Geometry: final body of the model. Coordinates: model frame, mm. Give positions to 0.01 mm unless a question says otherwise; leave off trailing zeros. Write each loop counter-clockwise with the first axis right and the second up, starting at its lowest first coordinate (ties: lowest second). Pieces come first, ordered by that corner, then holes. Notation, with made-up numbers: M -6,-28 L 34,-28 A25 cw 34,2 Z; hole C -25.5,-40 d2. An arc over 180 degrees is marked long. Use one line per item in the form item = value. Start each with the question number.
Item 1: Contact query for a flat-ended pin moving along its axis: P1, Ø5.5, axis at x = 0, y = 0, coming from the +Z side. Output: stop coordinate, or through.
Item 2: Section query A-A on x = 0. Return loops of the section in (y, z).
Item 3: Material intervals for line 1 along Y through (x, z) = (0, -0.7); line 2 along X through (y, z) = (80, -0.35); line 3 along X through (y, z) = (66, 0.75), sorted ascending. Write a range as from..to.
Item 4: Section query C-C on y = 30. Return loops of the section in (x, z), then the cut area to 3 significant figures.
Item 5: Section query B-B on z = 0.95. Return loops of the section in (x, y), then the cut area to 3 significant figures.
Autodesk Inventor part; units mm, degrees
ref_plane "YZ Plane" through (0, 0, 0) normal (1, 0, 0) x (0, 1, 0)
ref_plane "XZ Plane" through (0, 0, 0) normal (0, 1, 0) x (-1, 0, 0)
ref_plane "XY Plane" through (0, 0, 0) normal (0, 0, 1) x (1, 0, 0)
sketch "Sketch1" plane through (0, 0, 0) normal (0, 0, 1) x (1, 0, 0)
  circle A0 centre (0, 0) radius 6
  line L0 (0, 0) -> (0, 80) construction
  line L1 (6, 0) -> (6, 80)
  line L2 (-6, 80) -> (-6, 0)
  arc A1 (-6, 0) -> (6, 0) centre (0, 0) ccw
  arc A2 (6, 80) -> (-6, 80) centre (0, 80) ccw
  point P0 (0, 40)
  dimension "d0" = 12
  dimension "d1" = 12
  dimension "d2" = 80
extrude "Extrusion1" add sketch "Sketch1" along normal mid plane 2.8
sketch "Sketch2" plane through (0, 0, 1.4) normal (0, 0, 1) x (1, 0, 0)
  arc A0 (6, 80) -> (-6, 80) centre (0, 80) ccw construction
  arc A1 (-6, 0) -> (6, 0) centre (0, 0) ccw construction
  circle A2 centre (0, 0) radius 1.75
  circle A3 centre (0, 80) radius 1.75
  line L0 (-1.5, 64.9) -> (1.5, 64.9)
  line L1 (1.5, 64.9) -> (1.5, 70.1)
  line L2 (1.5, 70.1) -> (-1.5, 70.1)
  line L3 (-1.5, 70.1) -> (-1.5, 64.9)
  circle A4 centre (0, 30) radius 1.75
  line L4 (-1.5, 9.9) -> (1.5, 9.9)
  line L5 (1.5, 9.9) -> (1.5, 18.1)
  line L6 (1.5, 18.1) -> (-1.5, 18.1)
  line L7 (-1.5, 18.1) -> (-1.5, 9.9)
  point P0 (0, 9.9)
  point P1 (0, 64.9)
  point P2 (1.5, 14)
  point P3 (1.5, 67.5)
  dimension "d8" = 3.5
  dimension "d9" = 3.5
  dimension "d12" = 3
  dimension "d13" = 8.2
  dimension "d16" = 5.2
  dimension "d18" = 14
  dimension "d19" = 30
  dimension "d20" = 12.5
extrude "Extrusion2" cut sketch "Sketch2" against normal through all
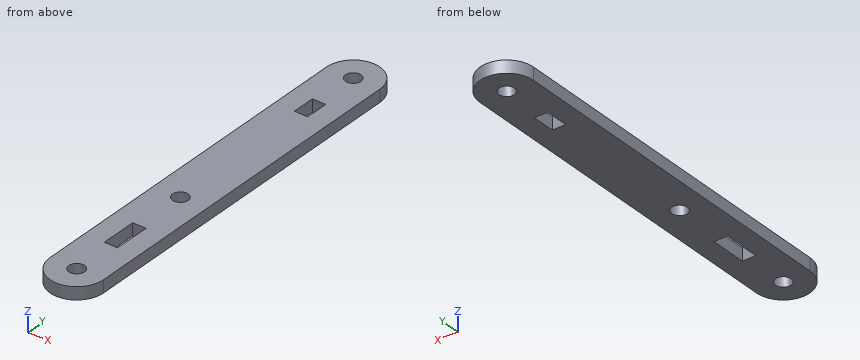
Answer sheet:
q1.P1 = 1.4
q2.outline = M -6,-1.4 L -1.75,-1.4 L -1.75,1.4 L -6,1.4 Z; M 1.75,-1.4 L 9.9,-1.4 L 9.9,1.4 L 1.75,1.4 Z; M 18.1,-1.4 L 28.25,-1.4 L 28.25,1.4 L 18.1,1.4 Z; M 31.75,-1.4 L 64.9,-1.4 L 64.9,1.4 L 31.75,1.4 Z; M 70.1,-1.4 L 78.25,-1.4 L 78.25,1.4 L 70.1,1.4 Z; M 81.75,-1.4 L 86,-1.4 L 86,1.4 L 81.75,1.4 Z
q3.line_1 = -6..-1.75, 1.75..9.9, 18.1..28.25, 31.75..64.9, 70.1..78.25, 81.75..86
q3.line_2 = -6..-1.75, 1.75..6
q3.line_3 = -6..-1.5, 1.5..6
q4.outline = M -6,-1.4 L -1.75,-1.4 L -1.75,1.4 L -6,1.4 Z; M 1.75,-1.4 L 6,-1.4 L 6,1.4 L 1.75,1.4 Z
q4.area = 23.8 mm2
q5.outline = M -6,0 A6 ccw 6,0 L 6,80 A6 ccw -6,80 Z; hole C 0,0 d3.5; hole C 0,30 d3.5; hole C 0,80 d3.5; hole M -1.5,9.9 L 1.5,9.9 L 1.5,18.1 L -1.5,18.1 Z; hole M -1.5,64.9 L 1.5,64.9 L 1.5,70.1 L -1.5,70.1 Z
q5.area = 1,000 mm2
